The figure shows three views and two pictorial views of one solid part (mm, origin at its lowest corner). Answer the questions. A direction names the side the tool comes from. Coordinates: 2 decimals unless noted, no trailing zeros. Write each loop counter-clockwise with the first axis right and the second up, starting at its lowest first coordinate (ties: lowest second). Pieces come first, ordered by that corner, then holes.
Item 1: Section B-B (z = 21) is taken. Give the vertices of the cut face in (x, y), then the cut area to 3 significant figures.
Item 2: A tool of negligible diameter and unlimited length cuts with its end or side. For the marked faces 1 and 2, from which of +Z, -Z, +X, -X, +Y, -Y can it reach the whole face along a straight path? Write none if from no direction.
Item 3: Straight lines are drawn through the part: probe 1 along Z at (x, y) = (21, 49.75); probe 2 along Y at (x, z) = (36, 17); probe 3 along Y at (x, z) = (32.5, 21.5). For each, find the intervals that lie inside material, in ascending order.
Item 4: Section C-C (x = 3.5) is taken. Give the vertices of the cut face in (y, z).
Item 5: Section A-A (y = 48) is taken. Give the vertices of the cut face in (x, z), then the cut area to 3 significant figures.
Item 6: Each of these flat-tipped pins is pushed along its axis until it touches: P1, Ø3, axis at x = 32, z = 37, coming from the +Y side; P2, Ø5, axis at x = 14, z = 26, coming from the +Y side; P3, Ø12, axis at y = 40.5, z = 9.5, coming from the -X side. Where does it stop, or does it pass through?
Item 7: Section D-D (y = 63.5) is taken. Give the vertices of the cut face in (x, z), then the cut area to 3 significant figures.
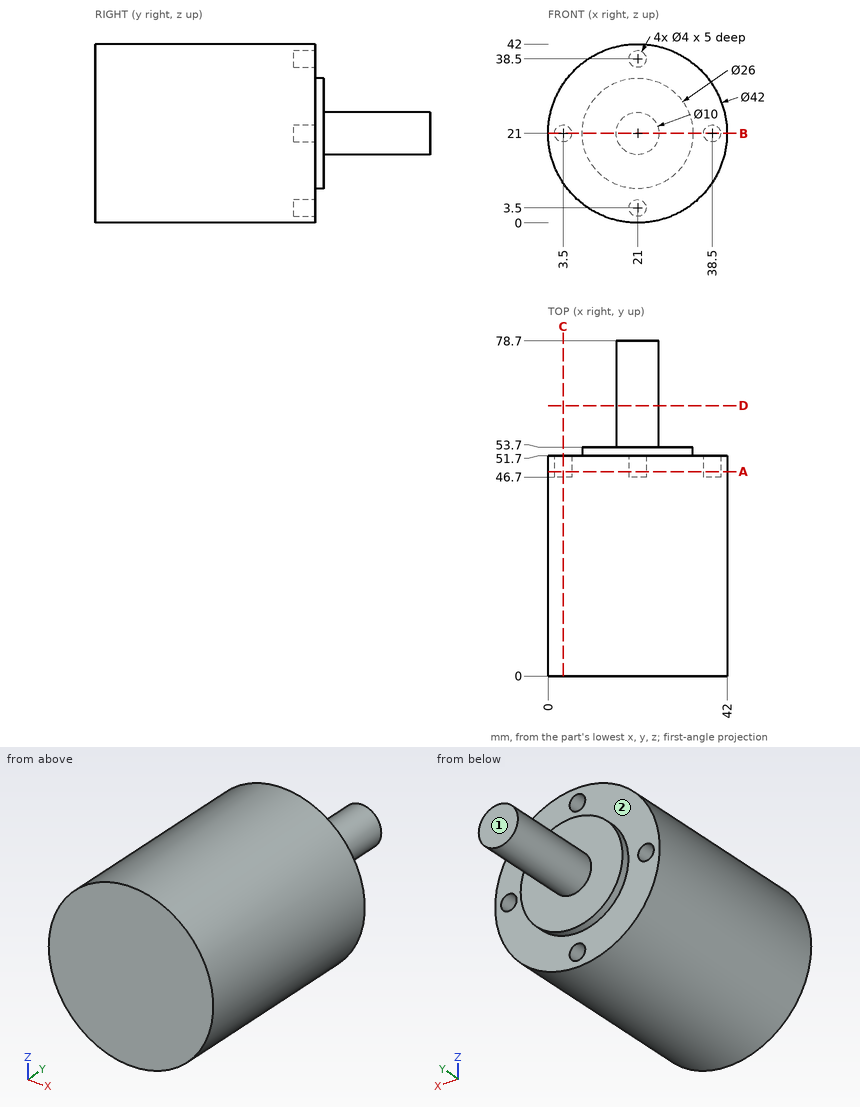
Established:
1. outline: (0, 0) - (42, 0) - (42, 51.7) - (40.5, 51.7) - (40.5, 46.7) - (36.5, 46.7) - (36.5, 51.7) - (34, 51.7) - (34, 53.7) - (26, 53.7) - (26, 78.7) - (16, 78.7) - (16, 53.7) - (8, 53.7) - (8, 51.7) - (5.5, 51.7) - (5.5, 46.7) - (1.5, 46.7) - (1.5, 51.7) - (0, 51.7) - close
1. area: 2,430 mm2
2. face 1: +Z, -Z, +X, -X, +Y
2. face 2: +Y
3. probe 1: z = 0 to 1.5, 5.5 to 36.5, 40.5 to 42
3. probe 2: y = 0 to 51.7
3. probe 3: y = 0 to 53.7
4. outline: (0, 9.39) - (51.7, 9.39) - (51.7, 19) - (46.7, 19) - (46.7, 23) - (51.7, 23) - (51.7, 32.61) - (0, 32.61) - close
5. outline: circle Ø42 at (21, 21); hole circle Ø4 at (3.5, 21); hole circle Ø4 at (21, 3.5); hole circle Ø4 at (21, 38.5); hole circle Ø4 at (38.5, 21)
5. area: 1,340 mm2
6. P1: stops at y = 51.7
6. P2: stops at y = 53.7
6. P3: stops at x = 0.73
7. outline: circle Ø10 at (21, 21)
7. area: 78.5 mm2
